from build123d import *

# Parameters (mm, degrees)
SKETCH1_R           = 1.5
SKETCH1_R_2         = 0.75
SKETCH1_R_3         = 1.25
SKETCH1_R_4         = 1
BOSS_EXTRUDE1_DEPTH = 5


with BuildPart() as part:
    # Sketch1 → Boss-Extrude1 (new body)
    with BuildSketch(Plane.XY):
        with BuildLine():
            Line((53.483314774, 4), (49.325917677, -2.222222222))
            ThreePointArc((49.325917677, -2.222222222), (46, -4), (42.674082323, -2.222222222))
            Line((42.674082323, -2.222222222), (38.516685226, 4))
            Line((38.516685226, 4), (20, 4))
            Line((20, 4), (20, 4.615103075))
            ThreePointArc((20, 4.615103075), (19.114133272, 6.743586222), (16.979706327, 7.615034435))
            Line((16.979706327, 7.615034435), (9.43588174, 7.56400263))
            ThreePointArc((9.43588174, 7.56400263), (6.909923235, 6.150450748), (6.754411009, 3.260050907))
            ThreePointArc((6.754411009, 3.260050907), (4.183258191, -6.224977984), (-5.570203117, -5.022234287))
            Line((-5.570203117, -5.022234287), (-8.426937489, -1.853805696))
            ThreePointArc((-8.426937489, -1.853805696), (-10.334596266, 1.25568183), (-11, 4.842506687))
            Line((-11, 4.842506687), (-11, 13))
            ThreePointArc((-11, 13), (-9.66809518, 15.980145652), (-6.559365945, 16.975656126))
            ThreePointArc((-6.559365945, 16.975656126), (19.092866868, 15.791235692), (44.685411632, 17.903474458))
            ThreePointArc((44.685411632, 17.903474458), (53.605257844, 13.812489287), (53.483314774, 4))
        make_face()
        Circle(SKETCH1_R, mode=Mode.SUBTRACT)
        with Locations((46, 0)):
            Circle(SKETCH1_R_2, mode=Mode.SUBTRACT)
        with Locations((46, 9)):
            Circle(SKETCH1_R_3, mode=Mode.SUBTRACT)
        with Locations((-7, 13)):
            Circle(SKETCH1_R_4, mode=Mode.SUBTRACT)
    extrude(amount=BOSS_EXTRUDE1_DEPTH)


solid = part.part
Build history of the part. All positions in model axes, mm. A direction names the side the tool comes from. Round coordinates to 2 decimals unless told otherwise and drop trailing zeros. Write each loop counter-clockwise with the first axis right and the second up, starting at its lowest first coordinate (ties: lowest second). Pieces come first, ordered by that corner, then holes. Notation, with made-up numbers: (6.5, -30) -> (56.5, -30) arc R7 cw to (56.5, -18) -> close; hole circle Ø7 at (54.5, 50.25). An arc over 180 degrees is marked (long way). Write item = value, one per line.
(1) Two-plate mould, pull along Y, no slides. Class faces 1 (the face through (40.62, 0.85, 2.46)), 2 (the face through (-7, 12, 2)), 3 (the face through (-11, 9, 2)), 4 (the face through (6.933, 6.186, 2.465)): pulls with the +Y half, pulls with the -Y half, needs draft (parallel to the pull), parting line crosses it, or undercut.
Answer:
face_1 = pulls with the -Y half
face_2 = undercut
face_3 = needs draft
face_4 = undercut
(2) Tool access for faces 5 (the face through (29, 4, 2)), 6 (the face through (-10.316, 1.208, 2.465)): list every direction of +Z, -Z, +X, -X, +Y, -Y with a clear straight run to the whole face (end or side of a thin tool).
Answer:
face_5 = +Z, -Z, -Y
face_6 = +Z, -Z, -X, -Y
(3) Band-saw the part on D-D (z = 2.1). Give the cut face in (x, y).
Answer:
outline = (-11, 4.84) arc R10 ccw to (-8.43, -1.85) -> (-5.57, -5.02) arc R7.5 ccw to (6.75, 3.26) arc R3 cw to (9.44, 7.56) -> (16.98, 7.62) arc R3 cw to (20, 4.62) -> (20, 4) -> (38.52, 4) -> (42.67, -2.22) arc R4 ccw to (49.33, -2.22) -> (53.48, 4) arc R9 ccw to (44.69, 17.9) arc R200 cw to (-6.56, 16.98) arc R4 ccw to (-11, 13) -> close; hole circle Ø2 at (-7, 13); hole circle Ø3 at (0, 0); hole circle Ø2.5 at (46, 9); hole circle Ø1.5 at (46, 0)
(4) Band-saw the part on B-B (y = 9). Give the cut face in (x, z), then the cut area to 4 significant figures.
Answer:
outline = (-11, 0) -> (44.75, 0) -> (44.75, 5) -> (-11, 5) -> close; (47.25, 0) -> (55, 0) -> (55, 5) -> (47.25, 5) -> close
area = 317.5 mm2
(5) Probe L1, parallel to Y at x = 46, z = 3.7; L2, parallel to X at y = 0.25, z = 0.7; L3, parallel to Y at x = 0, z = 1.65. List the from-to ranges inside material, lowest first.
Answer:
L1 = -4 to -0.75, 0.75 to 7.75, 10.25 to 18
L2 = -9.88 to -1.48, 1.48 to 7.5, 41.02 to 45.29, 46.71 to 50.98
L3 = -7.5 to -1.5, 1.5 to 16.36
(6) Flat gauge pins, fed straight in: pin 1 (2.5 mm diameter, centred on x = -7, y = 13, fed in from -Z); pin 2 (8 mm diameter, centred on x = 12.5, y = 3, fed in from -Z); pin 3 (1.5 mm diameter, centred on x = 32.5, z = 1.5, fed in from -Y); pin 4 (2 mm diameter, centred on x = 25, z = 2, fed in from +Y). Where does each tip first touch, or does it go through?
Answer:
pin_1 = 0
pin_2 = through
pin_3 = 4
pin_4 = 16.04
(7) Band-saw the part on C-C (y = 0). Give the cut face in (x, z), then the cut area to 3 significant figures.
Answer:
outline = (-9.75, 0) -> (-1.5, 0) -> (-1.5, 5) -> (-9.75, 5) -> close; (1.5, 0) -> (7.5, 0) -> (7.5, 5) -> (1.5, 5) -> close; (41.19, 0) -> (45.25, 0) -> (45.25, 5) -> (41.19, 5) -> close; (46.75, 0) -> (50.81, 0) -> (50.81, 5) -> (46.75, 5) -> close
area = 112 mm2
(8) Band-saw the part on A-A (x = 46). Give the cut face in (y, z).
Answer:
outline = (-4, 0) -> (-0.75, 0) -> (-0.75, 5) -> (-4, 5) -> close; (0.75, 0) -> (7.75, 0) -> (7.75, 5) -> (0.75, 5) -> close; (10.25, 0) -> (18, 0) -> (18, 5) -> (10.25, 5) -> close
